Job drawing, mm, ordinate dimensions from the low corner. One solid piece. Coordinates: 2 decimals unless noted, no trailing zeros. Loops run counter-clockwise (first coordinate to the right, second up) from the corner with the lowest first, then second, coordinate; pieces in that order, holes last. Notation, with made-up numbers: M 42.5,58.25 L 71.5,58.25 A29 cw 71.5,86.25 Z; hole C -10.75,27 d1. An arc over 180 degrees is marked long. Answer as a JSON object with one key per item and string values. Group by question number.
1. Drill centre lines: L1, parallel to X at y = 3.85, z = 69; L2, parallel to X at y = 1.3, z = 64.5; L3, parallel to Z at x = 7, y = 1.35. Where is each one in solid material? Low to high.
2. Drop flat-ended pins along their axis: pin 1 Ø1.3 at (x, y) = (40, 1.5) entering from +Z; pin 2 Ø2 at (y, z) = (2, 65.5) entering from -X; pin 3 Ø1.3 at (y, z) = (1, 10) entering from +X. Give the stop position or say it passes through.
3. Saw through at B-B on x = 25.4. Write the cut outline in (y, z) (1 decimal).
4. Saw through at A-A on y = 3.2. Write the cut outline in (x, z).
5. Saw through at D-D on x = 12. Write the cut outline in (y, z) (1 decimal), then the cut area to 3 significant figures.
6. Saw through at C-C on z = 10. Write the cut outline in (x, y) (1 decimal).
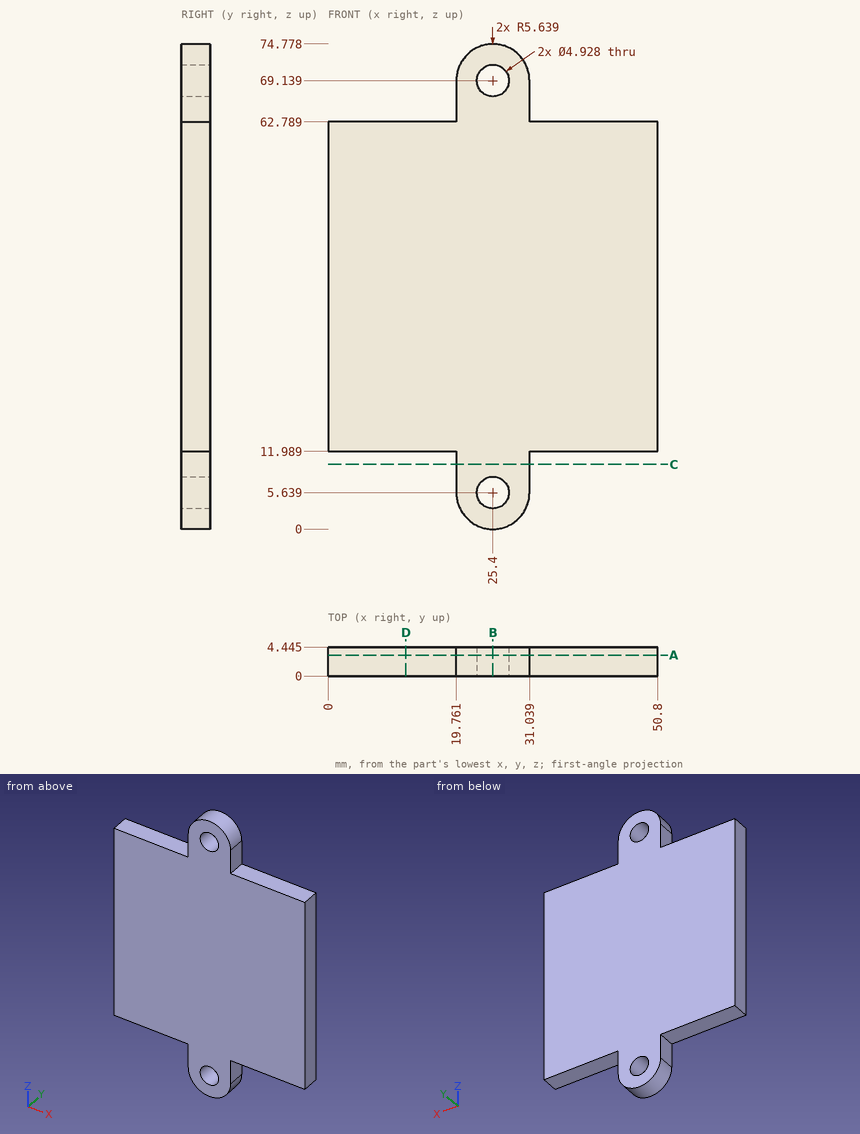
Outcome:
{
 "1": {"L1": "x = 19.76 to 22.94, 27.86 to 31.04", "L2": "x = 19.76 to 31.04", "L3": "z = 11.99 to 62.79"},
 "2": {"pin 1": "stops at z = 62.79", "pin 2": "stops at x = 19.76", "pin 3": "stops at x = 31.04"},
 "3": {"outline": "M 0,0 L 4.4,0 L 4.4,3.2 L 0,3.2 Z; M 0,8.1 L 4.4,8.1 L 4.4,66.7 L 0,66.7 Z; M 0,71.6 L 4.4,71.6 L 4.4,74.8 L 0,74.8 Z"},
 "4": {"outline": "M 0,11.99 L 19.76,11.99 L 19.76,5.64 A5.64 ccw 31.04,5.64 L 31.04,11.99 L 50.8,11.99 L 50.8,62.79 L 31.04,62.79 L 31.04,69.14 A5.64 ccw 19.76,69.14 L 19.76,62.79 L 0,62.79 Z; hole C 25.4,5.64 d4.93; hole C 25.4,69.14 d4.93"},
 "5": {"outline": "M 0,12 L 4.4,12 L 4.4,62.8 L 0,62.8 Z", "area": "226 mm²"},
 "6": {"outline": "M 19.8,0 L 31,0 L 31,4.4 L 19.8,4.4 Z"}
}
